Source: CAD feature listing. Evaluate the final solid. Frame: model axes, mm. A direction names the side the tool comes from. Round coordinates to 2 decimals unless told otherwise and drop trailing zeros. Loops run counter-clockwise (first coordinate to the right, second up) from the corner with the lowest first, then second, coordinate; pieces in that order, holes last.
(1) Set-up query: faces 1 (the conical face through (28.7, -4.96, 8.45)), 2 (the flat face through (10.5, 0.8, 9.462)). Return all of +Z, -Z, +X, -X, +Y, -Y with unobstructed straight access to the full face (end or side cutting, diameter ignored); none if empty.
(2) First-contact query: pin 1 Ø3 at (x, z) = (23, -3.5) entering from -Y; pin 2 Ø5 at (x, y) = (17, -4.5) entering from -Z; pin 3 Ø4.5 at (y, z) = (0, 0) entering from +X. Flat tips, straight axial feed; report the tip coordinate or a pass-through.
(3) Mould query, pull axis Z, two halves, no side actions, for faces 3 (the flat face through (30, -2, 0)), 4 (the flat face through (25, 0, -9.5)), 5 (the flat face through (25, 0, 9.5)), 6 (the cylindrical face through (24.17, 10.55, -0.01)). Classes: pulls with the +Z half, pulls with the -Z half, needs draft (parallel to the pull), parting line crosses it, or undercut.
(4) Section B-B, the plane x = 28.5. Return the cut outline in (y, z), plus the area to 3 significant figures.
(5) Section A-A, the plane x = 3. Return the cut outline in (y, z).
(6) Material intervals for probe 1 along X at (y, z) = (6.25, -7.75); probe 2 along Z at (x, y) = (15, 1.25); probe 3 along Y at (x, z) = (23, 1.5), sorted ascending.
```python
from build123d import *

# Parameters (mm, degrees)
ESQUISSE2_W             = 38
ESQUISSE2_H             = 38
ENL_V_MAT_EXTRU_1_DEPTH = 36
ESQUISSE3_W             = 3.666666666
ESQUISSE3_H             = 3.666666666
ENL_V_MAT_EXTRU_2_DEPTH = 0.038


with BuildPart() as part:
    # Esquisse1 → Révolution1 (revolve)
    with BuildSketch(Plane.XY, mode=Mode.PRIVATE) as r_volution1_sk:
        with BuildLine():
            Line((0.585, 1.75), (30, 1.75))
            Line((30, 1.75), (30, 7.6))
            ThreePointArc((30, 7.6), (32.507864279, 6.743550024), (33.967991826, 4.532008174))
            ThreePointArc((33.967991826, 4.532008174), (34.610930007, 3.281443073), (36, 3.5))
            ThreePointArc((36, 3.5), (34.242640687, 7.742640687), (30, 9.5))
            Line((30, 9.5), (29, 9.5))
            Line((29, 9.5), (25.833333333, 12.666666667))
            Line((25.833333333, 12.666666667), (20.5, 12.666666667))
            Line((20.5, 12.666666667), (20.5, 7.6))
            Line((20.5, 7.6), (13, 7.6))
            Line((13, 7.6), (13, 12.666666667))
            Line((13, 12.666666667), (8, 12.666666667))
            Line((8, 12.666666667), (8, 7.22))
            Line((8, 7.22), (6.4, 7.22))
            Line((6.4, 7.22), (5.741820693, 7.6))
            Line((5.741820693, 7.6), (0.8, 7.6))
            Line((0.8, 7.6), (0.8, 7.22))
            Line((0.8, 7.22), (0.585, 7.22))
            ThreePointArc((0.585, 7.22), (0.171342533, 7.048657467), (0, 6.635))
            Line((0, 6.635), (0, 2.335))
            ThreePointArc((0, 2.335), (0.171342533, 1.921342533), (0.585, 1.75))
        make_face()
    revolve(r_volution1_sk.sketch.rotate(Axis((36, 0, 0), (-1, 0, 0)), 90), axis=Axis((36, 0, 0), (-1, 0, 0)))

    # Esquisse2 → Enlèv. mat.-Extru.1 (cut)
    with BuildSketch(Plane(origin=(8, 0, 0), x_dir=(0, 0, -1), z_dir=(1, 0, 0))):
        Rectangle(ESQUISSE2_W, ESQUISSE2_H)
        with BuildLine():
            Line((-9.5, 4.588300339), (-9.5, -4.588300339))
            ThreePointArc((-9.5, -4.588300339), (-9.13656801, -5.275), (-8.723584654, -5.933091166))
            Line((-8.723584654, -5.933091166), (-0.776415346, -10.521391505))
            ThreePointArc((-0.776415346, -10.521391505), (0, -10.55), (0.776415346, -10.521391505))
            Line((0.776415346, -10.521391505), (8.723584654, -5.933091166))
            ThreePointArc((8.723584654, -5.933091166), (9.13656801, -5.275), (9.5, -4.588300339))
            Line((9.5, -4.588300339), (9.5, 4.588300339))
            ThreePointArc((9.5, 4.588300339), (9.13656801, 5.275), (8.723584654, 5.933091166))
            Line((8.723584654, 5.933091166), (0.776415346, 10.521391505))
            ThreePointArc((0.776415346, 10.521391505), (0, 10.55), (-0.776415346, 10.521391505))
            Line((-0.776415346, 10.521391505), (-8.723584654, 5.933091166))
            ThreePointArc((-8.723584654, 5.933091166), (-9.13656801, 5.275), (-9.5, 4.588300339))
        make_face(mode=Mode.SUBTRACT)
    extrude(amount=ENL_V_MAT_EXTRU_1_DEPTH, mode=Mode.SUBTRACT)

    # Esquisse3 → Enlèv. mat.-Extru.2 (cut)
    with BuildSketch(Plane.XY.offset(9.5)):
        with Locations((10.5, 0)):
            Rectangle(ESQUISSE3_W, ESQUISSE3_H)
        with BuildLine():
            Line((9.390432265, -1.243638701), (9.465872252, -1.139804467))
            ThreePointArc((9.465872252, -1.139804467), (10.23876211, -0.359563109), (9.735544583, -1.335732884))
            Line((9.735544583, -1.335732884), (9.660104596, -1.439567118))
            ThreePointArc((9.660104596, -1.439567118), (10.5, -1.666666667), (11.339895404, -1.439567118))
            Line((11.339895404, -1.439567118), (11.264455417, -1.335732884))
            ThreePointArc((11.264455417, -1.335732884), (10.76123789, -0.359563109), (11.534127748, -1.139804467))
            Line((11.534127748, -1.139804467), (11.609567735, -1.243638701))
            ThreePointArc((11.609567735, -1.243638701), (12.085094194, -0.515028324), (12.128651642, 0.353937293))
            Line((12.128651642, 0.353937293), (12.006587179, 0.314276144))
            ThreePointArc((12.006587179, 0.314276144), (10.922691785, 0.137340886), (11.903581514, 0.631294983))
            Line((11.903581514, 0.631294983), (12.025645977, 0.670956131))
            ThreePointArc((12.025645977, 0.670956131), (11.479642087, 1.348361657), (10.666666667, 1.658312395))
            Line((10.666666667, 1.658312395), (10.666666667, 1.529966223))
            ThreePointArc((10.666666667, 1.529966223), (10.5, 0.444444444), (10.333333333, 1.529966223))
            Line((10.333333333, 1.529966223), (10.333333333, 1.658312395))
            ThreePointArc((10.333333333, 1.658312395), (9.520357913, 1.348361657), (8.974354023, 0.670956131))
            Line((8.974354023, 0.670956131), (9.096418486, 0.631294983))
            ThreePointArc((9.096418486, 0.631294983), (10.077308215, 0.137340886), (8.993412821, 0.314276144))
            Line((8.993412821, 0.314276144), (8.871348358, 0.353937293))
            ThreePointArc((8.871348358, 0.353937293), (8.914905806, -0.515028324), (9.390432265, -1.243638701))
        make_face(mode=Mode.SUBTRACT)
    extrude(amount=-ENL_V_MAT_EXTRU_2_DEPTH, mode=Mode.SUBTRACT)


solid = part.part
```
Output values:
1. face 1: +Z, +X, -Y
1. face 2: +Z
2. pin 1: stops at y = -9.81
2. pin 2: stops at z = -7.33
2. pin 3: stops at x = 30
3. face 3: undercut
3. face 4: pulls with the -Z half
3. face 5: pulls with the +Z half
3. face 6: parting line crosses it
4. outline: (-9.79, -2.05) - (-6.67, -7.45) arc R10 ccw to (-3.12, -9.5) - (3.12, -9.5) arc R10 ccw to (6.67, -7.45) - (9.79, -2.05) arc R10 ccw to (9.79, 2.05) - (6.67, 7.45) arc R10 ccw to (3.12, 9.5) - (-3.12, 9.5) arc R10 ccw to (-6.67, 7.45) - (-9.79, 2.05) arc R10 ccw to start; hole circle Ø3.5 at (0, 0)
4. area: 292 mm2
5. outline: circle Ø15.2 at (0, 0); hole circle Ø3.5 at (0, 0)
6. probe 1: x = 8 to 13, 20.5 to 28.54
6. probe 2: z = -7.5 to -1.22, 1.22 to 7.5
6. probe 3: y = -10.1 to -0.9, 0.9 to 10.1
